from build123d import *

# Parameters (mm, degrees)
F1_W = 7.327596
F1_H = 4.832284


with BuildPart() as f2:
    # F2: sweep along a path in F0
    with BuildLine(Plane.XY) as f2_path:
        Line((0, 0), (20.490962, 0))
        ThreePointArc((20.490962, 0), (24.981091, -1.859872), (26.840962, -6.35))
        Line((26.840962, -6.35), (26.840962, -15.191156))
        ThreePointArc((26.840962, -15.191156), (24.981091, -19.681284), (20.490962, -21.541156))
        Line((20.490962, -21.541156), (0, -21.541156))
    # F1 (on Right) → F2 (sweep)
    with BuildSketch(Plane.YZ):
        with Locations((3.663798, 2.416142)):
            Rectangle(F1_W, F1_H)
    sweep(path=f2_path.line)


solid = f2.part
Check sheet for the modelled part. Datum: model origin and axes. Units: mm. A direction names the side the tool comes from. Round coordinates to 2 decimals unless told otherwise and drop trailing zeros. Loops run counter-clockwise (first coordinate to the right, second up) from the corner with the lowest first, then second, coordinate; pieces in that order, holes last. Notation, with made-up numbers: M 58,77.5 L 100,77.5 A10 cw 100,82.5 Z; hole C 37,25 d10. An arc over 180 degrees is marked long. One line per question, with ' | ' between items. Start each with the question number.
Item 1: Scan lines: probe 1 along Y at (x, z) = (4.5, 0.95); probe 2 along X at (y, z) = (-14.5, 3.85); probe 3 along Y at (x, z) = (24, 0.4). Record each from-to range of solid material in increasing order.
Item 2: Release check for a two-part mould opening along Y. For faces 3 (the face through (34.169, -11, 2)), 4 (the face through (30.056, 3.427, 2.45)), 5 (the face through (10, 0, 2)) record: released by +Y, released by -Y, zero draft, split by the parting line, or undercut.
Item 3: Section check B-B (z = 2.5). Record the boundary of the cut face in (x, y).
Item 4: Section check D-D (y = -13). Record the boundary of the cut face in (x, z), and give its area (3 significant figures).
Item 5: Gauge pin test, flat end, axial feed: pin 1 Ø6 at (x, y) = (15, 1) entering from -Z. Record the tip position at first contact, or that the pin passes through.
Item 6: Set-up check for faces 1 (the face through (29, -11, 4.832)), 2 (the face through (24.93, -1.81, 2.38)): record each of +Z, -Z, +X, -X, +Y, -Y from which the full face is reachable in a straight line by a thin tool's end or side.
Item 7: Section check A-A (x = 18). Record the boundary of the cut face in (y, z), and give its area (3 significant figures).
Item 8: Section check C-C (x = 22.5). Record the boundary of the cut face in (y, z), and give its area (3 significant figures).
Worked out:
1) probe 1: -28.87 to -21.54, 0 to 7.33 | probe 2: 26.84 to 34.17 | probe 3: -28.41 to -20.48, -1.06 to 6.87
2) face 3: zero draft | face 4: released by +Y | face 5: undercut
3) outline: M 0,-28.87 L 20.49,-28.87 A13.68 ccw 34.17,-15.19 L 34.17,-6.35 A13.68 ccw 20.49,7.33 L 0,7.33 L 0,0 L 20.49,0 A6.35 cw 26.84,-6.35 L 26.84,-15.19 A6.35 cw 20.49,-21.54 L 0,-21.54 Z
4) outline: M 26.84,0 L 34.17,0 L 34.17,4.83 L 26.84,4.83 Z | area: 35.4 mm^2
5) pin 1: z = 0
6) face 1: +Z, +X, -X, +Y, -Y | face 2: +Z, -Z, -X
7) outline: M -28.87,0 L -21.54,0 L -21.54,4.83 L -28.87,4.83 Z; M 0,0 L 7.33,0 L 7.33,4.83 L 0,4.83 Z | area: 70.8 mm^2
8) outline: M -28.72,0 L -21.21,0 L -21.21,4.83 L -28.72,4.83 Z; M -0.33,0 L 7.18,0 L 7.18,4.83 L -0.33,4.83 Z | area: 72.5 mm^2
